Input: part model. Units: mm. Frame: model coordinates. A direction names the side the tool comes from. Round coordinates to 2 decimals unless told otherwise and drop trailing zeros. Order: outer loops, then holes, each group sorted by start corner. A loop starts at its lowest first (then second) coordinate and runs counter-clockwise, first axis right, second up. Notation, with made-up numbers: (18, 28.5) -> (69, 28.5) arc R16 ccw to (69, 48.5) -> close; hole circle Ø4 at (-25, 73.5). An arc over 180 degrees is marked (long way). Use a Markdown table: item, result.
from build123d import *

# Parameters (mm, degrees)
BOSS_EXTRUDE1_DEPTH = 300
SKETCH3_R           = 2.25
CUT_EXTRUDE1_DEPTH  = 300
SKETCH6_R           = 2.25
CUT_EXTRUDE2_DEPTH  = 10
SKETCH7_R           = 1.85
CUT_EXTRUDE3_DEPTH  = 301.537152445


with BuildPart() as part:
    # Sketch1 → Boss-Extrude1 (new body)
    with BuildSketch(Plane(origin=(0, 0, 0), x_dir=(1, 0, 0), z_dir=(0, 1, 0))):
        Polygon((0, 0), (12.7, 0), (12.7, 3.18), (3.18, 3.18), (3.18, 12.7), (0, 12.7), align=None)
    extrude(amount=BOSS_EXTRUDE1_DEPTH)

    # Sketch3 → Cut-Extrude1 (cut)
    with BuildSketch(Plane(origin=(0, 0, -3.18), x_dir=(-1, 0, 0), z_dir=(0, 0, -1))):
        with Locations((-7.94, 275)):
            Circle(SKETCH3_R)
        with Locations((-7.94, 175)):
            Circle(SKETCH3_R)
        with Locations((-7.94, 75)):
            Circle(SKETCH3_R)
    extrude(amount=-CUT_EXTRUDE1_DEPTH, mode=Mode.SUBTRACT)

    # Sketch6 → Cut-Extrude2 (cut)
    with BuildSketch(Plane(origin=(3.18, 0, 0), x_dir=(0, 0, -1), z_dir=(1, 0, 0))):
        with Locations((7.94, 225)):
            Circle(SKETCH6_R)
        with Locations((7.94, 125)):
            Circle(SKETCH6_R)
        with Locations((7.94, 25)):
            Circle(SKETCH6_R)
    extrude(amount=-CUT_EXTRUDE2_DEPTH, mode=Mode.SUBTRACT)

    # Sketch7 → Cut-Extrude3 (cut, through all)
    with BuildSketch(Plane.XY):
        with Locations((7.94, 253.6)):
            Circle(SKETCH7_R)
    extrude(amount=-CUT_EXTRUDE3_DEPTH, mode=Mode.SUBTRACT)


solid = part.part
1) Contact query for flat-ended pins moving along their axis: P1, Ø2.5, axis at x = 7.94, y = 275, coming from the -Z side; P2, Ø1, axis at x = 8, y = 240, coming from the -Z side; P3, Ø5, axis at y = 180, z = -6, coming from the +X side. Output: stop coordinate, or through.
Answer key:
| item | result |
|---|---|
| P1 | passes through |
| P2 | stops at z = -3.18 |
| P3 | stops at x = 3.18 |
2) Set-up query: faces 1 (the face through (8, 148, -3.18)), 2 (the face through (0, 148, -6)). Return all of +Z, -Z, +X, -X, +Y, -Y with unobstructed straight access to the full face (end or side cutting, diameter ignored); none if empty.
Answer key:
| item | result |
|---|---|
| face 1 | -Z, +X, +Y, -Y |
| face 2 | +Z, -Z, -X, +Y, -Y |
3) Cut plane B-B on y = 35. Return loops of the section in (x, z), and give its area (3 significant figures).
Answer key:
| item | result |
|---|---|
| outline | (0, -12.7) -> (3.18, -12.7) -> (3.18, -3.18) -> (12.7, -3.18) -> (12.7, 0) -> (0, 0) -> close |
| area | 70.7 mm^2 |
4) Ray query, probe 1 along Y at (x, z) = (7.94, -1.9); probe 2 along Y at (x, z) = (1.85, -7.94); probe 3 along X at (y, z) = (175, -1.1). Return the intervals inside material, ascending.
Answer key:
| item | result |
|---|---|
| probe 1 | y = 0 to 72.75, 77.25 to 172.75, 177.25 to 251.75, 255.45 to 272.75, 277.25 to 300 |
| probe 2 | y = 0 to 22.75, 27.25 to 122.75, 127.25 to 222.75, 227.25 to 300 |
| probe 3 | x = 0 to 5.69, 10.19 to 12.7 |
5) Cut plane A-A on z = -7.94. Return loops of the section in (x, y), and give its area (3 significant figures).
Answer key:
| item | result |
|---|---|
| outline | (0, 0) -> (3.18, 0) -> (3.18, 22.75) -> (0, 22.75) -> close; (0, 27.25) -> (3.18, 27.25) -> (3.18, 122.75) -> (0, 122.75) -> close; (0, 127.25) -> (3.18, 127.25) -> (3.18, 222.75) -> (0, 222.75) -> close; (0, 227.25) -> (3.18, 227.25) -> (3.18, 300) -> (0, 300) -> close |
| area | 911 mm^2 |
